from build123d import *

# Parameters (mm, degrees)
SKETCH_1_W          = 20
SKETCH_1_H          = 7
SKETCH_1_W_2        = 50
EXTRUDE_1_DEPTH     = 39
CUT_EXTRUDE_1_DEPTH = 5
EXTRUDE_2_REACH     = 60.949
SKETCH_3_W          = 7
SKETCH_3_H          = 5
EXTRUDE_3_REACH     = 74.429
SKETCH_4_W          = 7
SKETCH_4_H          = 14
SKETCH_4_H_2        = 3.5
CUT_EXTRUDE_2_REACH = 78.059
SKETCH_5_W          = 18
SKETCH_5_H          = 6
SKETCH_6_W          = 23
SKETCH_6_H          = 14
EXTRUDE_4_DEPTH     = 8
EXTRUDE_5_DEPTH     = 2
EXTRUDE_6_DEPTH     = 6


with BuildPart() as part:
    # Эскиз1 → Бобышка-Вытянуть1 (new body)
    with BuildSketch(Plane.XY):
        with Locations((17, 31.5)):
            Rectangle(SKETCH_1_W, SKETCH_1_H)
        Polygon((0, 35), (0, 0), (7, 0), (7, 28), (7, 35), align=None)
        with Locations((25, -3.5)):
            Rectangle(SKETCH_1_W_2, SKETCH_1_H)
    extrude(amount=EXTRUDE_1_DEPTH)

    # Эскиз2 → Вырез-Вытянуть1 (cut)
    with BuildSketch(Plane(origin=(0, 35, 0), x_dir=(1, 0, 0), z_dir=(0, 1, 0))):
        with BuildLine():
            ThreePointArc((7, -15), (3.818019485, -16.318019485), (2.5, -19.5))
            Line((2.5, -19.5), (11.5, -19.5))
            ThreePointArc((11.5, -19.5), (10.181980515, -16.318019485), (7, -15))
        make_face()
        with BuildLine():
            Line((11.5, -19.5), (2.5, -19.5))
            ThreePointArc((2.5, -19.5), (3.818019485, -22.681980515), (7, -24))
            ThreePointArc((7, -24), (10.181980515, -22.681980515), (11.5, -19.5))
        make_face()
        with BuildLine():
            Line((0, -15), (0, -19.5))
            Line((0, -19.5), (2.5, -19.5))
            ThreePointArc((2.5, -19.5), (3.818019485, -16.318019485), (7, -15))
            Line((7, -15), (0, -15))
        make_face()
        with BuildLine():
            Line((2.5, -19.5), (0, -19.5))
            Line((0, -19.5), (0, -24))
            Line((0, -24), (7, -24))
            ThreePointArc((7, -24), (3.818019485, -22.681980515), (2.5, -19.5))
        make_face()
    extrude(amount=-CUT_EXTRUDE_1_DEPTH, mode=Mode.SUBTRACT)

    # Эскиз3 → Бобышка-Вытянуть2 (add, up to next)
    with BuildSketch(Plane(origin=(27, 0, 0), x_dir=(0, 0, -1), z_dir=(1, 0, 0)), mode=Mode.PRIVATE) as extrude_2_sk1:
        with Locations((-3.5, 25.5)):
            Rectangle(SKETCH_3_W, SKETCH_3_H)
    extrude_2_tool1 = extrude(extrude_2_sk1.sketch, amount=-EXTRUDE_2_REACH, mode=Mode.PRIVATE) - part.part
    add(extrude_2_tool1.solids().sort_by_distance((27, 25.5, 3.5))[0])

    # Бобышка-Вытянуть3: up to this face of the body (flat: up to its plane)
    extrude_3_end = Plane(part.part.faces().sort_by_distance((0, 13.47740113, 19.5))[0])
    # Эскиз4 → Бобышка-Вытянуть3 (add, up to the picked face)
    with BuildSketch(Plane(origin=(50, 0, 0), x_dir=(0, 0, -1), z_dir=(1, 0, 0)), mode=Mode.PRIVATE) as extrude_3_sk1:
        with Locations((-35.5, -3.5)):
            Rectangle(SKETCH_4_W, SKETCH_4_H)
    extrude_3_tool1 = split(extrude(extrude_3_sk1.sketch, amount=-EXTRUDE_3_REACH, mode=Mode.PRIVATE), bisect_by=extrude_3_end, keep=Keep.BOTH, mode=Mode.PRIVATE)
    # Эскиз4 → Бобышка-Вытянуть3 (add, up to the picked face)
    with BuildSketch(Plane(origin=(50, 0, 0), x_dir=(0, 0, -1), z_dir=(1, 0, 0)), mode=Mode.PRIVATE) as extrude_3_sk2:
        with Locations((-9.5, -8.75)):
            Rectangle(SKETCH_4_W, SKETCH_4_H_2)
    extrude_3_tool2 = split(extrude(extrude_3_sk2.sketch, amount=-EXTRUDE_3_REACH, mode=Mode.PRIVATE), bisect_by=extrude_3_end, keep=Keep.BOTH, mode=Mode.PRIVATE)
    add(extrude_3_tool1.solids().sort_by(Axis((50, -3.5, 35.5), (-1, 0, 0)))[0])
    add(extrude_3_tool2.solids().sort_by(Axis((50, -8.75, 9.5), (-1, 0, 0)))[0])

    # Эскиз5 → Вырез-Вытянуть2 (cut, up to next)
    with BuildSketch(Plane.XZ.offset(7), mode=Mode.PRIVATE) as cut_extrude_2_sk1:
        with Locations((25, 3)):
            Rectangle(SKETCH_5_W, SKETCH_5_H)
    cut_extrude_2_tool1 = extrude(cut_extrude_2_sk1.sketch, amount=-CUT_EXTRUDE_2_REACH, mode=Mode.PRIVATE) & part.part
    add(cut_extrude_2_tool1.solids().sort_by_distance((25, -7, 3))[0], mode=Mode.SUBTRACT)

    # Эскиз6 → Бобышка-Вытянуть4 (add)
    with BuildSketch(Plane.XY.offset(39)):
        with Locations((28.5, -3.5)):
            Rectangle(SKETCH_6_W, SKETCH_6_H)
    extrude(amount=EXTRUDE_4_DEPTH)

    # Эскиз7 → Бобышка-Вытянуть5 (add)
    with BuildSketch(Plane.ZY):
        Polygon((39, -10.5), (39, 35), (24, 35), (24, 30), (15, 30), (15, 35), (0, 35), (0, -7), (6, -7), (6, -10.5), (13, -10.5), (13, -7), (32, -7), (32, -10.5), align=None)
    extrude(amount=EXTRUDE_5_DEPTH)

    # Эскиз8 → Бобышка-Вытянуть6 (add)
    with BuildSketch(Plane(origin=(0, 3.5, 0), x_dir=(1, 0, 0), z_dir=(0, 1, 0))):
        Polygon((7, -32), (7, -39), (17, -39), (17, -47), (40, -47), (40, -39), (50, -39), (50, -32), align=None)
    extrude(amount=EXTRUDE_6_DEPTH)


solid = part.part
Could you check a few things on this model? Use its own coordinates, in mm. A direction names the side the tool comes from. Give positions to 0.01 mm unless a question says otherwise; leave off trailing zeros. Order: outer loops, then holes, each group sorted by start corner. A loop starts at its lowest first (then second) coordinate and runs counter-clockwise, first axis right, second up.
1. For pin 1 (1 mm diameter, centred on x = 9.5, y = 11.5, fed in from -Z); pin 2 (10 mm diameter, centred on y = 30, z = 34.5, fed in from +X); pin 3 (5 mm diameter, centred on x = 19.5, z = 18, fed in from -Y); pin 4 (2.5 mm diameter, centred on x = 21, y = 25, fed in from +Z), each with a flat end and sliding along its axis, tell me the tip position at first contact or that it passes through.
Answers below:
pin 1: passes through
pin 2: stops at x = 27
pin 3: stops at y = -7
pin 4: stops at z = 7
2. Which directions (+Z, -Z, +X, -X, +Y, -Y) give clear straight access to the entire face, cutting with the end or side of a thin tool? Please do faces 4 (the flat face through (5, 30, 20)), 5 (the flat face through (27, 30, 15)), 6 (the flat face through (24, -9, 13)).
Answers below:
face 4: -X, +Y
face 5: +Z, -Z, +X, +Y
face 6: +X, -X, -Y
3. Thinking about a two-plate mould opening in Z: for faces 1 (the flat face through (24, -9, 32)), 2 (the flat face through (45, -1, 39)), 3 (the flat face through (13, 35, 20)), which applies, +Z half, -Z half, draft (parallel to the pull), parting line (faces both ways), or undercut?
Answers below:
face 1: undercut
face 2: +Z half
face 3: draft
4. Suppose I cut it at A-A (x = 23.5). Write out the boundary of the cut face in (y, z).
Answers below:
outline: (-10.5, 6) - (0, 6) - (0, 32) - (9.5, 32) - (9.5, 47) - (-10.5, 47) - (-10.5, 32) - (-7, 32) - (-7, 13) - (-10.5, 13) - close; (23, 0) - (35, 0) - (35, 39) - (28, 39) - (28, 7) - (23, 7) - close
5. Suppose I cut it at D-D (x = 4). Write out the boundary of the cut face in (y, z), plus the area to 3 significant figures.
Answers below:
outline: (-10.5, 6) - (-7, 6) - (-7, 0) - (35, 0) - (35, 15) - (30, 15) - (30, 24) - (35, 24) - (35, 39) - (-10.5, 39) - (-10.5, 32) - (-7, 32) - (-7, 13) - (-10.5, 13) - close
area: 1,640 mm2
6. Suppose I cut it at C-C (z = 37). Write out the boundary of the cut face in (x, y), plus the area to 3 significant figures.
Answers below:
outline: (-2, -10.5) - (50, -10.5) - (50, 9.5) - (7, 9.5) - (7, 28) - (27, 28) - (27, 35) - (-2, 35) - close
area: 1,410 mm2
7. I need wall thicknesses on L1, parallel to Y at x = 22, z = 16.5; L2, parallel to Z at x = 4.5, y = 31; L3, parallel to Z at x = 32, y = 3.5. Which ranges of each line are inside material? Lowest first, please.
Answers below:
L1: y = -7 to 0, 28 to 35
L2: z = 0 to 15, 24 to 39
L3: z = 32 to 47
8. Suppose I cut it at B-B (y = 3.5). Write out the boundary of the cut face in (x, z).
Answers below:
outline: (-2, 0) - (7, 0) - (7, 32) - (50, 32) - (50, 39) - (40, 39) - (40, 47) - (17, 47) - (17, 39) - (-2, 39) - close
